from build123d import *

# Parameters (mm, degrees)
SKETCH1_W                   = 80
SKETCH1_H                   = 80
BOSS_EXTRUDE1_DEPTH         = 3
SKETCH2_W                   = 17.5
SKETCH2_H                   = 17.5
BOSS_EXTRUDE2_DEPTH         = 10
SKETCH3_W                   = 14.3
SKETCH3_H                   = 14.3
CUT_EXTRUDE1_DEPTH          = 10
TAP_DRILL_FOR_M3X0_5_TAP1_D = 2.5
TAP_DRILL_FOR_M3X0_5_TAP2_D = 2.5
MIRROR2_COPY_1_SKETCH_W     = 17.5
MIRROR2_COPY_1_SKETCH_H     = 17.5
MIRROR2_COPY_1_DEPTH        = 10
MIRROR2_COPY_2_SKETCH_W     = 14.3
MIRROR2_COPY_2_SKETCH_H     = 14.3
MIRROR2_COPY_2_DEPTH        = 10
MIRROR2_COPY_3_D            = 2.5
MIRROR2_COPY_4_D            = 2.5


with BuildPart() as part:
    # Sketch1 → Boss-Extrude1 (new body)
    with BuildSketch(Plane(origin=(0, 0, 0), x_dir=(1, 0, 0), z_dir=(0, 1, 0))):
        Rectangle(SKETCH1_W, SKETCH1_H)
    extrude(amount=BOSS_EXTRUDE1_DEPTH)

    # Sketch2 → Boss-Extrude2 (add)
    with BuildSketch(Plane(origin=(0, 3, 0), x_dir=(1, 0, 0), z_dir=(0, 1, 0))):
        with Locations((-18.75, 18.75)):
            Rectangle(SKETCH2_W, SKETCH2_H)
    boss_extrude2 = extrude(amount=BOSS_EXTRUDE2_DEPTH)

    # Sketch3 → Cut-Extrude1 (cut)
    with BuildSketch(Plane(origin=(0, 13, 0), x_dir=(1, 0, 0), z_dir=(0, 1, 0))):
        with Locations((-18.75, 18.75)):
            Rectangle(SKETCH3_W, SKETCH3_H)
    cut_extrude1 = extrude(amount=-CUT_EXTRUDE1_DEPTH, mode=Mode.SUBTRACT)

    # Tap Drill for M3x0.5 Tap1 (through all)
    with Locations(Plane.XY.offset(-10)):
        with Locations((-18.75, 8)):
            tap_drill_for_m3x0_5_tap1 = Hole(TAP_DRILL_FOR_M3X0_5_TAP1_D / 2)

    # Tap Drill for M3x0.5 Tap2 (through all)
    with Locations(Plane.ZY.offset(27.5)):
        with Locations((-18.75, 8)):
            tap_drill_for_m3x0_5_tap2 = Hole(TAP_DRILL_FOR_M3X0_5_TAP2_D / 2)

    # Mirror1: Boss-Extrude2, Cut-Extrude1, Tap Drill for M3x0.5 Tap1, Tap Drill for M3x0.5 Tap2 across plane
    add(boss_extrude2.mirror(Plane.ZY))
    add(cut_extrude1.mirror(Plane.ZY), mode=Mode.SUBTRACT)
    add(tap_drill_for_m3x0_5_tap1.mirror(Plane.ZY), mode=Mode.SUBTRACT)
    add(tap_drill_for_m3x0_5_tap2.mirror(Plane.ZY), mode=Mode.SUBTRACT)

    # Mirror2: Boss-Extrude2, Cut-Extrude1, Tap Drill for M3x0.5 Tap1, Tap Drill for M3x0.5 Tap2 across plane
    add(boss_extrude2.mirror(Plane.XY))
    add(cut_extrude1.mirror(Plane.XY), mode=Mode.SUBTRACT)
    add(tap_drill_for_m3x0_5_tap1.mirror(Plane.XY), mode=Mode.SUBTRACT)
    add(tap_drill_for_m3x0_5_tap2.mirror(Plane.XY), mode=Mode.SUBTRACT)

    # Mirror2 copy 1 sketch → Mirror2 copy 1 (add)
    with BuildSketch(Plane(origin=(0, 3, 0), x_dir=(-1, 0, 0), z_dir=(0, 1, 0))):
        with Locations((-18.75, 18.75)):
            Rectangle(MIRROR2_COPY_1_SKETCH_W, MIRROR2_COPY_1_SKETCH_H)
    extrude(amount=MIRROR2_COPY_1_DEPTH)

    # Mirror2 copy 2 sketch → Mirror2 copy 2 (cut)
    with BuildSketch(Plane(origin=(0, 13, 0), x_dir=(-1, 0, 0), z_dir=(0, 1, 0))):
        with Locations((-18.75, 18.75)):
            Rectangle(MIRROR2_COPY_2_SKETCH_W, MIRROR2_COPY_2_SKETCH_H)
    extrude(amount=-MIRROR2_COPY_2_DEPTH, mode=Mode.SUBTRACT)

    # Mirror2 copy 3 (through all)
    with Locations(Plane(origin=(0, 0, 10), x_dir=(-1, 0, 0), z_dir=(0, 0, -1))):
        with Locations((-18.75, 8)):
            Hole(MIRROR2_COPY_3_D / 2)

    # Mirror2 copy 4 (through all)
    with Locations(Plane(origin=(27.5, 0, 0), x_dir=(0, 0, -1), z_dir=(1, 0, 0))):
        with Locations((-18.75, 8)):
            Hole(MIRROR2_COPY_4_D / 2)


solid = part.part
Input: part model. Units: mm. Frame: model coordinates. A direction names the side the tool comes from. Give positions to 0.01 mm unless a question says otherwise; leave off trailing zeros. Write each loop counter-clockwise with the first axis right and the second up, starting at its lowest first coordinate (ties: lowest second). Pieces come first, ordered by that corner, then holes. Notation, with made-up numbers: M 87,80 L 92,80 A18 cw 92,89 Z; hole C 68.5,29.25 d3. An arc over 180 degrees is marked long. Write item = value, one per line. Start each with the question number.
1) Cut plane A-A on z = -15. Return the cut outline in (x, y), then the cut area to 3 significant figures.
2) Cut plane B-B on x = 23.5. Return the cut outline in (y, z).
3) Draft query along Z for faces 1 (the flat face through (25.9, 8, -17)), 2 (the cylindrical face through (20, 8, -11)), 3 (the flat face through (17, 8, 27.5)). Return one class per face: +Z half, -Z half, draft (parallel to the pull), parting line (faces both ways), or undercut.
4) First-contact query: pin 1 Ø1.5 at (x, y) = (20, 7) entering from -Z; pin 2 Ø3 at (y, z) = (8, 18.75) entering from +X; pin 3 Ø5 at (y, z) = (4.5, 23.5) entering from +X; pin 4 Ø2 at (y, z) = (8, -18.75) entering from +X. Flat tips, straight axial feed; report the tip coordinate or a pass-through.
5) Material intervals for line 1 along X through (y, z) = (5, -22); line 2 along Z through (x, y) = (11, 11.75); line 3 along Y through (x, z) = (-18.75, 10.95), sorted ascending. Write a range as [from, to].
6) Cut plane C-C on y = 8. Count the separate pieces of the cut face and the enclosed holes in it, then the cut area to 3 significant figures.
7) Reachability of faces 4 (the flat face through (17, 8, -27.5)), 5 (the cylindrical face through (27, 8, 20)), 6 (the flat face through (-17, 8, -25.9)), 7 (the flat face through (-17, 8, 27.5)), 8 (the flat face through (17, 8, 10)) from +Z, -Z, +X, -X, +Y, -Y: full face, straight path, thin tool, end or side. Return the list, or none.
Solved:
q1.outline = M -40,0 L 40,0 L 40,3 L 27.5,3 L 27.5,13 L 25.9,13 L 25.9,3 L 11.6,3 L 11.6,13 L 10,13 L 10,3 L -10,3 L -10,13 L -11.6,13 L -11.6,3 L -25.9,3 L -25.9,13 L -27.5,13 L -27.5,3 L -40,3 Z
q1.area = 304 mm2
q2.outline = M 0,-40 L 3,-40 L 3,-27.5 L 13,-27.5 L 13,-25.9 L 3,-25.9 L 3,-11.6 L 13,-11.6 L 13,-10 L 3,-10 L 3,10 L 13,10 L 13,11.6 L 3,11.6 L 3,25.9 L 13,25.9 L 13,27.5 L 3,27.5 L 3,40 L 0,40 Z
q3.face_1 = undercut
q3.face_2 = draft
q3.face_3 = +Z half
q4.pin_1 = -27.5
q4.pin_2 = 27.5
q4.pin_3 = 40
q4.pin_4 = through
q5.line_1 = [-27.5, -25.9], [-11.6, -10], [10, 11.6], [25.9, 27.5]
q5.line_2 = [-27.5, -10], [10, 27.5]
q5.line_3 = [0, 6.75], [9.25, 13]
q6.separate_pieces = 16
q6.enclosed_holes = 0
q6.area = 343 mm2
q7.face_4 = -Z, +X, -X, +Y
q7.face_5 = +X, -X
q7.face_6 = +Y
q7.face_7 = +Z, +X, -X, +Y
q7.face_8 = +X, -X, +Y
